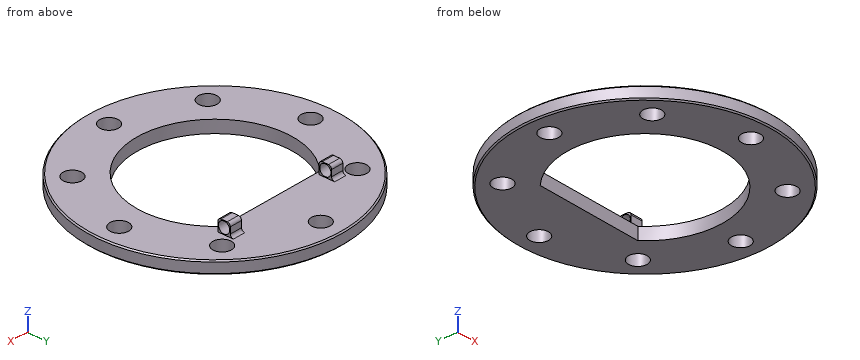
from build123d import *

# Parameters (mm, degrees)
SKETCH1_R                      = 205
SKETCH1_R_2                    = 15
BOSS_EXTRUDE1_DEPTH            = 20
CHAMFER1_SIZE                  = 2
CUT_EXTRUDE1_DEPTH             = 20
SKETCH4_W                      = 20
SKETCH4_H                      = 20
BOSS_EXTRUDE2_DEPTH            = 20
CUT_EXTRUDE3_REACH             = 294.66
SKETCH5_R                      = 9
CUT_EXTRUDE3_DIRECTION_2_REACH = 294.66
FILLET1_R                      = 5


with BuildPart() as part:
    # Sketch1 → Boss-Extrude1 (new body)
    with BuildSketch(Plane.XY):
        Circle(SKETCH1_R)
        with Locations((0, 170)):
            Circle(SKETCH1_R_2, mode=Mode.SUBTRACT)
        with Locations((120.208152802, 120.208152802)):
            Circle(SKETCH1_R_2, mode=Mode.SUBTRACT)
        with Locations((170, 0)):
            Circle(SKETCH1_R_2, mode=Mode.SUBTRACT)
        with Locations((120.208152802, -120.208152802)):
            Circle(SKETCH1_R_2, mode=Mode.SUBTRACT)
        with Locations((0, -170)):
            Circle(SKETCH1_R_2, mode=Mode.SUBTRACT)
        with Locations((-120.208152802, -120.208152802)):
            Circle(SKETCH1_R_2, mode=Mode.SUBTRACT)
        with Locations((-170, 0)):
            Circle(SKETCH1_R_2, mode=Mode.SUBTRACT)
        with Locations((-120.208152802, 120.208152802)):
            Circle(SKETCH1_R_2, mode=Mode.SUBTRACT)
    extrude(amount=BOSS_EXTRUDE1_DEPTH)

    # Chamfer1
    chamfer1_edges = [part.edges().sort_by_distance(p)[0] for p in [
        (-205, 0, 0),
        (-205, 0, 20),
    ]]
    chamfer(chamfer1_edges, length=CHAMFER1_SIZE)

    # Sketch2 → Cut-Extrude1 (cut)
    with BuildSketch(Plane.XY.offset(20)):
        with BuildLine():
            Line((-86.746757864, 90), (86.746757864, 90))
            ThreePointArc((86.746757864, 90), (0, -125), (-86.746757864, 90))
        make_face()
    extrude(amount=-CUT_EXTRUDE1_DEPTH, mode=Mode.SUBTRACT)

    # Sketch4 → Boss-Extrude2 (add)
    with BuildSketch(Plane.XY.offset(20)):
        with Locations((-90, 105)):
            Rectangle(SKETCH4_W, SKETCH4_H)
        with Locations((90, 105)):
            Rectangle(SKETCH4_W, SKETCH4_H)
    extrude(amount=BOSS_EXTRUDE2_DEPTH)

    # Cut-Extrude3: up to this face of the body (flat: up to its plane)
    cut_extrude3_end = Plane(part.part.faces().sort_by_distance((-100, 105, 30))[0])
    # Sketch5 → Cut-Extrude3 (cut, up to the picked face)
    with BuildSketch(Plane(origin=(0, 0, 0), x_dir=(0, 0, -1), z_dir=(1, 0, 0)), mode=Mode.PRIVATE) as cut_extrude3_sk1:
        with Locations((-30, 105)):
            Circle(SKETCH5_R)
    cut_extrude3_tool1 = split(extrude(cut_extrude3_sk1.sketch, amount=-CUT_EXTRUDE3_REACH, mode=Mode.PRIVATE), bisect_by=cut_extrude3_end, keep=Keep.BOTH, mode=Mode.PRIVATE)
    add(cut_extrude3_tool1.solids().sort_by(Axis((0, 105, 30), (-1, 0, 0)))[0], mode=Mode.SUBTRACT)

    # Cut-Extrude3 direction 2: up to this face of the body (flat: up to its plane)
    cut_extrude3_direction_2_end = Plane(part.part.faces().sort_by_distance((100, 105, 30))[0])
    # Sketch5 → Cut-Extrude3 direction 2 (cut, up to the picked face)
    with BuildSketch(Plane(origin=(0, 0, 0), x_dir=(0, 0, -1), z_dir=(1, 0, 0)), mode=Mode.PRIVATE) as cut_extrude3_direction_2_sk1:
        with Locations((-30, 105)):
            Circle(SKETCH5_R)
    cut_extrude3_direction_2_tool1 = split(extrude(cut_extrude3_direction_2_sk1.sketch, amount=CUT_EXTRUDE3_DIRECTION_2_REACH, mode=Mode.PRIVATE), bisect_by=cut_extrude3_direction_2_end, keep=Keep.BOTH, mode=Mode.PRIVATE)
    add(cut_extrude3_direction_2_tool1.solids().sort_by(Axis((0, 105, 30), (1, 0, 0)))[0], mode=Mode.SUBTRACT)

    # Fillet1
    fillet1_edges = [part.edges().sort_by_distance(p)[0] for p in [
        (-90, 115, 20),
        (-90, 95, 40),
        (-90, 115, 40),
        (90, 115, 20),
        (90, 115, 40),
        (90, 95, 40),
    ]]
    fillet(fillet1_edges, radius=FILLET1_R)


solid = part.part
Geometry check sheet. Reference: the model listing, model coordinates, mm. Give positions to 0.01 mm unless a question says otherwise; leave off trailing zeros. Loops run counter-clockwise (first coordinate to the right, second up) from the corner with the lowest first, then second, coordinate; pieces in that order, holes last. Notation, with made-up numbers: M 52.5,-1.75 L 90.5,-1.75 A23 ccw 90.5,13.25 Z; hole C -16,36.25 d3. An arc over 180 degrees is marked long. Write each question's results on one line, items separated by ' | '.
1) Gauge pin test, flat ends, axial feed: pin 1 (14.5 mm diameter, centred on y = 105, z = 30, fed in from -X); pin 2 (23.5 mm diameter, centred on y = 105, z = 30, fed in from -X); pin 3 (22 mm diameter, centred on y = 105.5, z = 32, fed in from -X); pin 4 (12 mm diameter, centred on x = 39, z = 8, fed in from +Y). Record the tip position at first contact, or that the pin passes through.
Answers follow:
pin 1: through | pin 2: x = -177.39 | pin 3: x = -100 | pin 4: y = 202.33
2) Thickness scan on line 1 (Y direction, x = 0, z = 5.25); line 2 (Y direction, x = 114, z = 8); line 3 (Z direction, x = 118.5, y = 101.5). Record the ranges inside material, lowest first.
Answers follow:
line 1: -205 to -185, -155 to -125, 90 to 155, 185 to 205 | line 2: -170.38 to -133.86, -106.55 to -51.27, 51.27 to 106.55, 133.86 to 170.38 | line 3: 0 to 20
3) Section check A-A, the plane z = 30. Record the boundary of the cut face in (x, y), plus the area to 3 significant figures.
Answers follow:
outline: M -100,95 L -80,95 L -80,96 L -100,96 Z; M -100,114 L -80,114 L -80,115 L -100,115 Z; M 80,95 L 100,95 L 100,96 L 80,96 Z; M 80,114 L 100,114 L 100,115 L 80,115 Z | area: 80.0 mm2
4) Section check B-B, the plane z = 8. Count the separate pieces of the cut face and the enclosed holes in it, plus the area to 3 significant figures.
Answers follow:
separate pieces: 1 | enclosed holes: 9 | area: 81,500 mm2
